Read the model definition and answer for the solid it produces. Units are mm, in the model's axes. A direction names the side the tool comes from. Coordinates: 2 decimals unless noted, no trailing zeros. Order: outer loops, then holes, each group sorted by start corner. A loop starts at its lowest first (then second) coordinate and runs counter-clockwise, first axis right, second up. Notation, with made-up numbers: M 30,-27 L 86,-27 A28 ccw 86,-6 Z; hole C -12.5,77.5 d11. An arc over 180 degrees is marked long. Use a Markdown table: item, result. Add a question column.
1) Find section B-B on z = 0. Write down the section's boundary in (x, y) (3 decimals), plus the area to 3 significant figures.
2) For faces 4 (the face through (16, -6, -3.175)), 5 (the face through (12.511, -11.567, 0.044)), 6 (the face through (4.7, -3.18, 0.14)), determine the directions among +Z, -Z, +X, -X, +Y, -Y from which every point of the face is accessible in a straight line to the end or side of a thin tool.
3) Find section D-D on z = 1.5. Write down the section's boundary in (x, y) (3 decimals).
4) Find the intervals of material crossed by probe 1 along X at (y, z) = (-6.35, 2.5) (3 decimals); probe 2 along Y at (x, z) = (12.75, 2); probe 3 along Z at (x, y) = (3, -6.5), in increasing order. Write a range as [from, to].
5) Find section A-A on y = -6.35. Write down the section's boundary in (x, z) (3 decimals), plus the area to 3 significant figures.
6) Find section C-C on x = 17.5. Write down the section's boundary in (y, z) (3 decimals).
7) Each of these flat-tipped pins is pushed along its axis until it touches: pin 1 Ø3 at (x, y) = (14.5, -5) entering from +Z; pin 2 Ø1.9 at (y, z) = (-7, -1) entering from -X (3 decimals); pin 3 Ø5.5 at (x, y) = (15.57, -6.35) entering from +Z (3 decimals). Where does it stop, or does it pass through?
8) The mould has two halves that part along Z. Classify faces 1 (the face through (11, -10, 6.35)), 2 (the face through (11, 0, 0)), 3 (the face through (9.525, -6, 0)): released by +Z, released by -Z, zero draft, split by the parting line, or undercut.
from build123d import *

# Parameters (mm, degrees)
SKETCH3_W                      = 21.924187445
SKETCH3_H                      = 19.837641971
BOSS_EXTRUDE1_DEPTH            = 6.35
SKETCH4_R                      = 3.175
CUT_EXTRUDE1_DEPTH             = 9.525
SKETCH5_R                      = 3.175
CUT_EXTRUDE5_DEPTH             = 9.525
CUT_EXTRUDE5_DIRECTION_2_REACH = 27.174
SKETCH6_R                      = 3.175
CUT_EXTRUDE6_DEPTH             = 9.525


with BuildPart() as part:
    # Sketch3 → Boss-Extrude1 (new, symmetric)
    with BuildSketch(Plane.XY):
        with Locations((10.962093723, -9.918820986)):
            Rectangle(SKETCH3_W, SKETCH3_H)
    extrude(amount=BOSS_EXTRUDE1_DEPTH, both=True)

    # Sketch4 → Cut-Extrude1 (cut)
    with BuildSketch(Plane.ZY):
        with Locations(Location((0, -6.35, 0), (0, 0, 270))):
            Circle(SKETCH4_R)
    extrude(amount=-CUT_EXTRUDE1_DEPTH, mode=Mode.SUBTRACT)

    # Sketch5 → Cut-Extrude5 (cut)
    with BuildSketch(Plane(origin=(7.787093723, -19.837641971, 0), x_dir=(-0.8660254037844382, 0.500000000000001, 0), z_dir=(-0.500000000000001, -0.8660254037844382, 0))):
        with Locations(Location((0, 0, 0), (0, 0, 180))):
            Circle(SKETCH5_R)
    extrude(amount=-CUT_EXTRUDE5_DEPTH, mode=Mode.SUBTRACT)

    # Sketch5 → Cut-Extrude5 direction 2 (cut, up to next)
    with BuildSketch(Plane(origin=(7.787093723, -19.837641971, 0), x_dir=(-0.8660254037844382, 0.500000000000001, 0), z_dir=(-0.500000000000001, -0.8660254037844382, 0)), mode=Mode.PRIVATE) as cut_extrude5_direction_2_sk1:
        with Locations(Location((0, 0, 0), (0, 0, 180))):
            Circle(SKETCH5_R)
    cut_extrude5_direction_2_tool1 = extrude(cut_extrude5_direction_2_sk1.sketch, amount=CUT_EXTRUDE5_DIRECTION_2_REACH, mode=Mode.PRIVATE) & part.part
    add(cut_extrude5_direction_2_tool1.solids().sort_by_distance((7.787094, -19.837642, 0))[0], mode=Mode.SUBTRACT)

    # Sketch6 → Cut-Extrude6 (cut)
    with BuildSketch(Plane(origin=(0, 0, 6.35), x_dir=(-1, 0, 0), z_dir=(0, 0, -1))):
        with Locations(Location((-15.574187445, -6.35, 0), (0, 0, 180))):
            Circle(SKETCH6_R)
    extrude(amount=CUT_EXTRUDE6_DEPTH, mode=Mode.SUBTRACT)


solid = part.part
Check result:
| question | item | result |
|---|---|---|
| 1 | outline | M 0,-19.838 L 4.121,-19.838 L 9.8,-10.001 L 15.299,-13.176 L 11.453,-19.838 L 21.924,-19.838 L 21.924,0 L 0,0 L 0,-3.175 L 9.525,-3.175 L 9.525,-9.525 L 0,-9.525 Z; hole C 15.574,-6.35 d6.35 |
| 1 | area | 282 mm2 |
| 2 | face 4 | +Z |
| 2 | face 5 | none |
| 2 | face 6 | -X |
| 3 | outline | M 0,-19.838 L 4.556,-19.838 L 10.126,-10.19 L 14.973,-12.988 L 11.018,-19.838 L 21.924,-19.838 L 21.924,0 L 0,0 L 0,-3.552 L 9.525,-3.552 L 9.525,-9.148 L 0,-9.148 Z; hole C 15.574,-6.35 d6.35 |
| 4 | probe 1 | x = [9.525, 12.399], [18.749, 21.924] |
| 4 | probe 2 | y = [-19.84, -16.17], [-11.7, -7.8], [-4.9, 0] |
| 4 | probe 3 | z = [-6.35, -3.17], [3.17, 6.35] |
| 5 | outline | M 0,-6.35 L 21.924,-6.35 L 21.924,6.35 L 18.749,6.35 L 18.749,-3.175 L 12.399,-3.175 L 12.399,6.35 L 0,6.35 L 0,3.175 L 9.525,3.175 L 9.525,-3.175 L 0,-3.175 Z |
| 5 | area | 157 mm2 |
| 6 | outline | M -19.838,-6.35 L 0,-6.35 L 0,6.35 L -3.826,6.35 L -3.826,-3.175 L -8.874,-3.175 L -8.874,6.35 L -19.838,6.35 Z |
| 7 | pin 1 | stops at z = 6.35 |
| 7 | pin 2 | stops at x = 9.525 |
| 7 | pin 3 | stops at z = -3.175 |
| 8 | face 1 | released by +Z |
| 8 | face 2 | zero draft |
| 8 | face 3 | undercut |
